```python
from build123d import *

# Parameters (mm, degrees)
F5_DEPTH  = 20
F6_SIZE   = 1.5
F7_SIZE   = 1.5
F11_DEPTH = 2.7510001


# Not quite as in the source:
# - a feature names something its author has since deleted; it is built from what else it names


with BuildPart() as f5:
    # F4 (on Front) → F5 (new body)
    with BuildSketch(Plane.XZ):
        with BuildLine():
            ThreePointArc((1.75, 4.3620522693), (3.0269919036, 3.5954582483), (4, 2.4677925359))
            Line((4, 2.4677925359), (4, 7.4677925359))
            Line((4, 7.4677925359), (-4, 7.4677925359))
            Line((-4, 7.4677925359), (-4, 2.4677925359))
            ThreePointArc((-4, 2.4677925359), (-3.0269919036, 3.5954582483), (-1.75, 4.3620522693))
            Line((-1.75, 4.3620522693), (-1.75, 5.2177925359))
            ThreePointArc((-1.75, 5.2177925359), (0, 6.9677925359), (1.75, 5.2177925359))
            Line((1.75, 5.2177925359), (1.75, 4.3620522693))
        make_face()
        with BuildLine():
            ThreePointArc((-1.75, 4.3620522693), (0, 4.7), (1.75, 4.3620522693))
            Line((1.75, 4.3620522693), (1.75, 5.2177925359))
            ThreePointArc((1.75, 5.2177925359), (0, 6.9677925359), (-1.75, 5.2177925359))
            Line((-1.75, 5.2177925359), (-1.75, 4.3620522693))
        make_face()
    extrude(amount=-F5_DEPTH)

    # F6
    f6_edges = [f5.edges().sort_by_distance(p)[0] for p in [
        (-4, 10, 7.467793),
        (4, 10, 7.467793),
    ]]
    chamfer(f6_edges, length=F6_SIZE)

    # F7
    f7_edges = [f5.edges().sort_by_distance(p)[0] for p in [
        (0, 20, 7.467793),
    ]]
    chamfer(f7_edges, length=F7_SIZE)

    # F9 (on offset) → F10 (revolve, cut)
    with BuildSketch(Plane.XY.offset(5.2177925359)):
        with BuildLine():
            Line((-1.75, 11.25), (-1.75, 0))
            Line((-1.75, 0), (0, 0))
            Line((0, 0), (0, 13))
            ThreePointArc((0, 13), (-1.2374368671, 12.4874368671), (-1.75, 11.25))
        make_face()
    revolve(axis=Axis((0, 6.5, 5.2177925359), (0, 1, 0)), mode=Mode.SUBTRACT)

    # F9 (on offset) → F11 (cut, through all)
    with BuildSketch(Plane.XY.offset(5.2177925359)):
        with BuildLine():
            Line((0, 13), (0, 0))
            Line((0, 0), (1.75, 0))
            Line((1.75, 0), (1.75, 11.25))
            ThreePointArc((1.75, 11.25), (1.2374368671, 12.4874368671), (0, 13))
        make_face()
        with BuildLine():
            Line((-1.75, 11.25), (-1.75, 0))
            Line((-1.75, 0), (0, 0))
            Line((0, 0), (0, 13))
            ThreePointArc((0, 13), (-1.2374368671, 12.4874368671), (-1.75, 11.25))
        make_face()
    extrude(amount=-F11_DEPTH, mode=Mode.SUBTRACT)


solid = f5.part
```
The listing builds one solid part. Answer for the finished solid, in the listing's coordinates (mm). A direction names the side the tool comes from. Coordinates: 2 decimals unless noted, no trailing zeros. Write each loop counter-clockwise with the first axis right and the second up, starting at its lowest first coordinate (ties: lowest second). Pieces come first, ordered by that corner, then holes. Notation, with made-up numbers: M 85.5,-20 L 137.5,-20 A26 cw 137.5,14 Z; hole C 78,24 d9. An arc over 180 degrees is marked long. Use a Markdown table: item, result. Add a question column.
1. Section A-A (z = 2.9) is taken. Give the vertices of the cut face in (x, y).
2. For a pull along X with two mould halves and no side action, classify faces 3 (the flat face through (-1.75, 6, 5)), 4 (the flat face through (0.06, 19.24, 6.73)), 5 (the flat face through (4, 10, 4)), 6 (the cylindrical face through (-0.038, 5.546, 6.967)) as +X half, -X half, draft (parallel to the pull), parting line (faces both ways), or undercut.
3. Which of the six approach directions +Z, -Z, +X, -X, +Y, -Y give full straight-line access (tool end or side, diameter ignored) to faces 1 (the flat face through (1.75, 6, 5)), 2 (the flat face through (0, 9, 7.468))?
4. Section C-C (z = 4.9) is taken. Give the vertices of the cut face in (x, y).
5. Straight lines are drawn through the part: line 1 along X through (y, z) = (4.75, 3.25); line 2 along X through (y, z) = (5.5, 3.85); line 3 along Z through (x, y) = (1.5, 18). For each, find the intervals that lie inside material, in ascending order. Write a range as [from, to].
6. Section B-B (y = 14.5) is taken. Give the vertices of the cut face in (x, z).
7. Section D-D (x = -1.5) is taken. Give the vertices of the cut face in (y, z), plus the area to 3 significant figures.
8. Given P1, Ø1.5, axis at x = 1.5, y = 3.5, coming from the -Z side, flat-ended and moving along its own axis, determine where the tip first touches the part or whether it passes through.
Data:
| question | item | result |
|---|---|---|
| 1 | outline | M -4,0 L -3.7,0 L -3.7,20 L -4,20 Z; M 3.7,0 L 4,0 L 4,20 L 3.7,20 Z |
| 2 | face 3 | undercut |
| 2 | face 4 | draft |
| 2 | face 5 | +X half |
| 2 | face 6 | undercut |
| 3 | face 1 | -Z, -Y |
| 3 | face 2 | +Z, +X, -X, +Y, -Y |
| 4 | outline | M -4,0 L -1.75,0 L -1.75,11.25 A1.75 cw 1.75,11.25 L 1.75,0 L 4,0 L 4,20 L -4,20 Z |
| 5 | line 1 | x = [-4, -3.4], [3.4, 4] |
| 5 | line 2 | x = [-4, -2.7], [2.7, 4] |
| 5 | line 3 | z = [4.45, 7.47] |
| 6 | outline | M -4,2.47 A4.7 cw 4,2.47 L 4,5.97 L 2.5,7.47 L -2.5,7.47 L -4,5.97 Z |
| 7 | outline | M 0,6.12 L 11.25,6.12 A0.9 cw 12.15,5.22 L 12.15,4.45 L 20,4.45 L 20,5.97 L 18.5,7.47 L 0,7.47 Z |
| 7 | area | 39.1 mm2 |
| 8 | P1 | stops at z = 4.13 |
